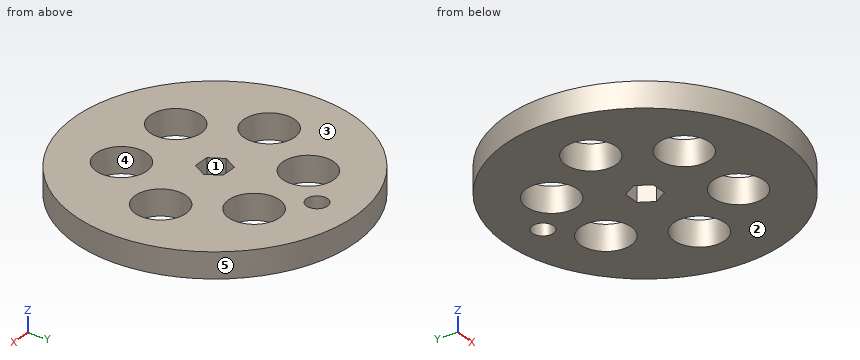
Autodesk Inventor part; units mm, degrees
ref_plane "YZ Plane" through (0, 0, 0) normal (1, 0, 0) x (0, 1, 0)
ref_plane "XZ Plane" through (0, 0, 0) normal (0, 1, 0) x (-1, 0, 0)
ref_plane "XY Plane" through (0, 0, 0) normal (0, 0, 1) x (1, 0, 0)
sketch "Sketch1" plane through (0, 0, 0) normal (0, 0, 1) x (1, 0, 0)
  circle A0 centre (0, 0) radius 69.85
  line L0 (7.9189, 0) -> (3.9595, -6.858)
  line L1 (3.9595, -6.858) -> (-3.9595, -6.858)
  line L2 (-3.9595, -6.858) -> (-7.9189, 0)
  line L3 (-7.9189, 0) -> (-3.9595, 6.858)
  line L4 (-3.9595, 6.858) -> (3.9595, 6.858)
  line L5 (3.9595, 6.858) -> (7.9189, 0)
  circle A1 centre (0, 50.8) radius 5.2705
  dimension "d0" = 139.7
  dimension "d1" = 13.716
  dimension "d2" = 10.541
  dimension "d5" = 50.8
extrude "Extrusion1" add sketch "Sketch1" along normal mid plane 12.7
sketch "Sketch2" plane through (0, 0, 6.35) normal (0, 0, 1) x (1, 0, 0)
  circle A0 centre (-38.1, 0) radius 12.7
  circle A1 centre (-19.05, -32.9956) radius 12.7
  circle A2 centre (19.05, -32.9956) radius 12.7
  circle A3 centre (38.1, 0) radius 12.7
  circle A4 centre (19.05, 32.9956) radius 12.7
  circle A5 centre (-19.05, 32.9956) radius 12.7
  point P0 (0, 0)
  dimension "d6" = 25.4
  dimension "d7" = 38.1
  dimension "d10" = 360
extrude "Extrusion2" cut sketch "Sketch2" against normal through all
properties part number "driveForPiston"
The model under review builds one solid part; all positions refer to its coordinate system, in mm. Face numbers are marked on the shaded views. A direction names the side the tool comes from. Coordinates: 2 decimals unless noted, no trailing zeros. Loops run counter-clockwise (first coordinate to the right, second up) from the corner with the lowest first, then second, coordinate; pieces in that order, holes last. Notation, with made-up numbers: (-8.75, 68) -> (17.25, 68) arc R18 cw to (17.25, 83) -> close; hole circle Ø6 at (15, 84). An arc over 180 degrees is marked (long way). Use a Markdown table: item, result. Add a question column.
1. Add section A-A on x = 0. Write out the cut boundary in (y, z), plus the area to 3 significant figures.
2. Draft analysis for pull direction X (two halves, no side actions). For the marked faces 3, 4 and 5, state which applies: pulls with the +X half, pulls with the -X half, needs draft (parallel to the pull), parting line crosses it, or undercut.
3. Add section C-C on y = -26.5. Write out the cut boundary in (x, z), plus the area to 3 significant figures.
4. Machinability: for the marked faces 1 and 2, which of the approach directions +Z, -Z, +X, -X, +Y, -Y give a long, thin tool a straight path to every point of the face, cutting with its end or side? Answer none if there is none.
5. Clearance check with flat-ended pins moving along their axes: pin 1 Ø1 at (x, z) = (46, 5) entering from +Y; pin 2 Ø1.5 at (y, z) = (-13.5, 0) entering from +X; pin 3 Ø6 at (y, z) = (-12.5, -3.5) entering from +X; pin 4 Ø10 at (x, y) = (46.5, -4) entering from +Z. State where each tip first meets the part, or that it passes through.
6. Add section B-B on x = -38.1. Write out the cut boundary in (y, z).
7. To check wall thickness, follow line 1 (X direction, y = -1, z = 2.5); line 2 (Y direction, x = 19.05, z = 0); line 3 (Y direction, x = -1, z = 4.5). State the ranges of each line that lie inside material, in increasing order.
8. Add section D-D on z = 4.5. Give the number of separate pieces and of enclosed holes in the cut face, plus the area to 3 significant figures.
Returned:
| question | item | result |
|---|---|---|
| 1 | outline | (-69.85, -6.35) -> (-6.86, -6.35) -> (-6.86, 6.35) -> (-69.85, 6.35) -> close; (6.86, -6.35) -> (45.53, -6.35) -> (45.53, 6.35) -> (6.86, 6.35) -> close; (56.07, -6.35) -> (69.85, -6.35) -> (69.85, 6.35) -> (56.07, 6.35) -> close |
| 1 | area | 1,470 mm² |
| 2 | face 3 | needs draft |
| 2 | face 4 | undercut |
| 2 | face 5 | parting line crosses it |
| 3 | outline | (-64.63, -6.35) -> (-29.96, -6.35) -> (-29.96, 6.35) -> (-64.63, 6.35) -> close; (-8.14, -6.35) -> (8.14, -6.35) -> (8.14, 6.35) -> (-8.14, 6.35) -> close; (29.96, -6.35) -> (64.63, -6.35) -> (64.63, 6.35) -> (29.96, 6.35) -> close |
| 3 | area | 1,090 mm² |
| 4 | face 1 | +Z, -Z |
| 4 | face 2 | -Z, +X, -X, +Y, -Y |
| 5 | pin 1 | stops at y = 53 |
| 5 | pin 2 | stops at x = 68.68 |
| 5 | pin 3 | stops at x = 69.2 |
| 5 | pin 4 | stops at z = 6.35 |
| 6 | outline | (-58.54, -6.35) -> (-12.7, -6.35) -> (-12.7, 6.35) -> (-58.54, 6.35) -> close; (12.7, -6.35) -> (58.54, -6.35) -> (58.54, 6.35) -> (12.7, 6.35) -> close |
| 7 | line 1 | x = -69.84 to -50.76, -25.44 to -7.34, 7.34 to 25.44, 50.76 to 69.84 |
| 7 | line 2 | y = -67.2 to -45.7, -20.3 to 20.3, 45.7 to 67.2 |
| 7 | line 3 | y = -69.84 to -6.86, 6.86 to 45.63, 55.97 to 69.84 |
| 8 | separate pieces | 1 |
| 8 | enclosed holes | 8 |
| 8 | area | 12,000 mm² |
